Autodesk Inventor part; units mm, degrees
ref_plane "YZ Plane" through (0, 0, 0) normal (1, 0, 0) x (0, 1, 0)
ref_plane "XZ Plane" through (0, 0, 0) normal (0, 1, 0) x (-1, 0, 0)
ref_plane "XY Plane" through (0, 0, 0) normal (0, 0, 1) x (1, 0, 0)
sketch "Sketch1" plane through (0, 0, 0) normal (1, 0, 0) x (0, 1, 0)
  circle A0 centre (0, 0) radius 4.7625
  line L0 (0, 0) -> (-63.5, 0) construction
  circle A1 centre (0, 0) radius 19.05
  line L1 (-5.715, 18.1725) -> (-63.5, 0)
  line L2 (-63.5, 0) -> (-63.5, -114.3)
  circle A2 centre (0, 0) radius 76.2 construction
  line L3 (-63.5, -114.3) -> (-28.575, -114.3)
  line L4 (-28.575, -114.3) -> (-28.575, -69.85)
  line L5 (-28.575, -69.85) -> (-63.5, -49.686)
  line L6 (-28.575, -69.85) -> (15.24, -11.43)
  line L7 (-39.6531, -63.4541) -> (-5.6963, -18.1784)
  line L8 (-53.975, -9.525) -> (-53.975, -55.1853)
  line L9 (-33.3375, -78.0989) -> (-63.5, -60.6846)
  line L10 (-33.3375, -78.0989) -> (-33.3375, -106.3625)
  line L11 (-33.3375, -106.3625) -> (-57.15, -106.3625)
  line L12 (-57.15, -106.3625) -> (-57.15, -64.3507)
  line L13 (-53.975, -9.525) -> (-52.0847, -9.525)
  line L14 (-52.0847, -9.525) -> (-16.4978, -9.525)
  line L15 (-63.5, 0) -> (-28.575, 0)
  line L16 (-28.575, 0) -> (-28.575, 25.4) construction
  line L17 (-28.575, 25.4) -> (-63.5, 25.4) construction
  line L18 (-63.5, 25.4) -> (-63.5, 0)
  line L19 (-28.575, 0) -> (-63.5, 25.4)
  point P0 (-39.1181, 7.6677)
  dimension "d0" = 9.525
  dimension "d1" = 63.5
  dimension "d2" = 38.1
  dimension "d3" = 114.3
  dimension "d4" = 152.4
  dimension "d5" = 34.925
  dimension "d6" = 44.45
  dimension "d7" = 60
  dimension "d9" = 12.7
  dimension "d10" = 9.525
  dimension "d11" = 9.525
  dimension "d12" = 7.9375
  dimension "d13" = 6.35
  dimension "d14" = 4.7625
  dimension "d17" = 9.525
  dimension "d19" = 34.925
  dimension "d20" = 25.4
extrude "Extrusion1" add sketch "Sketch1" along normal blind 4.7625 contours A1 | A1 L14 L13 L8 L5 L2 L15 L19 L1 | L6 L5 L7 A1 | L19 L15 L1 | L1 L18 L19 | L4 L3 L2 L5
fillet "Fillet1" radius 6.35 10 edges at (2.3813, -5.6963, -18.1784) (2.3813, -16.4978, -9.525) (2.3813, -39.6531, -63.4541) (2.3813, -53.975, -9.525) (2.3813, -53.975, -55.1853) (2.3813, -57.15, -64.3507) (2.3813, -33.3375, -78.0989) (2.3813, -33.3375, -106.3625) (2.3813, -57.15, -106.3625) (2.3813, -28.575, -69.85)
fillet "Fillet2" radius 6.35 2 edges at (2.3813, -63.5, 25.4) (2.3813, -39.1181, 7.6677)
sketch "Sketch2" plane through (4.7625, 0, 0) normal (1, 0, 0) x (0, 0, -1)
  circle A0 centre (0, 0) radius 4.7625
  circle A1 centre (0, 0) radius 11.1125
  dimension "d24" = 22.225
equation "\"d9\" = d8"
properties part number "Upright" material "Aluminum 6061"
Here's how the part is built. I have some questions about the finished solid (model axes, mm). A direction names the side the tool comes from. Give positions to 0.01 mm unless a question says otherwise; leave off trailing zeros. Order: outer loops, then holes, each group sorted by start corner. A loop starts at its lowest first (then second) coordinate and runs counter-clockwise, first axis right, second up. Notation, with made-up numbers: (-33, 75) -> (14, 75) arc R15 ccw to (14, 92) -> close; hole circle Ø10 at (-3, 7). An arc over 180 degrees is marked (long way). Use a Markdown table: item, result. Add a question column.
Item 1: Imagine slicing it at A-A on z = 0. Please give me the cut outline in (x, y).
Item 2: I need wall thicknesses on line 1 (Z direction, x = 2.6, y = -45) (1 decimal); line 2 (Z direction, x = 3.05, y = -34) (3 decimals); line 3 (Z direction, x = 2.3, y = -24.5) (3 decimals). Which ranges of each line are inside material? Lowest first, please.
Item 3: Imagine slicing it at D-D on y = -49. Please give me the cut outline in (x, z).
Item 4: Imagine slicing it at C-C on y = 0. Please give me the cut outline in (x, z).
Item 5: For faces 5 (the face through (2.41, -55.34, -104.45)), 6 (the face through (2.35, -47.48, 13.75)), which set-ups out of +Z, -Z, +X, -X, +Y, -Y let a thin tool reach every point of the face, with its end or its side?
Item 6: If we mould it in two halves opening along Y, with no side actions, what happens to faces 1 (the face through (2, -33.338, -91)), 2 (the face through (2.415, -34.165, -78.63)), 3 (the face through (2, -63.5, -50)), 4 (the face through (0, -14, -32))? For each: pulls with the +Y half, pulls with the -Y half, needs draft (parallel to the pull), parting line crosses it, or undercut.
Item 7: Imagine slicing it at B-B on x = 3. Give the number of separate pieces and of enclosed holes in the cut face, plus the area to 3 significant figures.
Item 8: Will this pin go through, and if not, where does the flat tip stop? pin 1 (2.5 mm diameter, centred on x = 3.5, y = -44, fed in from +Z).
Data:
| question | item | result |
|---|---|---|
| 1 | outline | (0, -63.5) -> (4.76, -63.5) -> (4.76, -4.76) -> (0, -4.76) -> close; (0, 4.76) -> (4.76, 4.76) -> (4.76, 19.05) -> (0, 19.05) -> close |
| 2 | line 1 | z = -114.3 to -106.4, -71.4 to -60.4, -9.5 to 11.9 |
| 2 | line 2 | z = -114.3 to -102.836, -78.941 to -55.917, -9.525 to 9.277 |
| 2 | line 3 | z = -64.417 to -43.25, -9.525 to 12.265 |
| 3 | outline | (0, -114.3) -> (4.76, -114.3) -> (4.76, -106.36) -> (0, -106.36) -> close; (0, -69.26) -> (4.76, -69.26) -> (4.76, -58.06) -> (0, -58.06) -> close; (0, -9.68) -> (4.76, -9.68) -> (4.76, 14.85) -> (0, 14.85) -> close |
| 4 | outline | (0, -31.75) -> (4.76, -31.75) -> (4.76, -4.76) -> (0, -4.76) -> close; (0, 4.76) -> (4.76, 4.76) -> (4.76, 19.05) -> (0, 19.05) -> close |
| 5 | face 5 | +X, -X |
| 5 | face 6 | +Z, +X, -X |
| 6 | face 1 | undercut |
| 6 | face 2 | undercut |
| 6 | face 3 | pulls with the -Y half |
| 6 | face 4 | needs draft |
| 7 | separate pieces | 1 |
| 7 | enclosed holes | 3 |
| 7 | area | 4,450 mm² |
| 8 | pin 1 | stops at z = 12.13 |
